Geometry check sheet. Reference: the model listing, model coordinates, mm. A direction names the side the tool comes from. Round coordinates to 2 decimals unless told otherwise and drop trailing zeros. Order: outer loops, then holes, each group sorted by start corner. A loop starts at its lowest first (then second) coordinate and runs counter-clockwise, first axis right, second up. Notation, with made-up numbers: (-11.5, 71) - (-1.5, 71) arc R5 ccw to (-1.5, 75) - close; hole circle Ø1 at (70, 58.25). An arc over 180 degrees is marked (long way). Return JSON: item names as keys, results as strings. Group by question number.
Q1. Gauge pin test, flat ends, axial feed: pin 1 Ø0.6 at (y, z) = (-6.5, 0.5) entering from +X; pin 2 Ø0.5 at (x, z) = (2.5, 1.5) entering from +Y; pin 3 Ø0.8 at (y, z) = (1, 1.5) entering from +X. Record the tip position at first contact, or that the pin passes through.
Q2. Sectioned sample at D-D, the plane x = -6.5. Record the cut outline in (y, z).
Q3. Material ranges on line 1 along Y through (x, z) = (0, 0.8); line 2 along Y through (x, z) = (-11, 0.6) (3 decimals); line 3 along Y through (x, z) = (-5, 1.6), recorded low to high.
Q4. Sectioned sample at C-C, the plane y = 0. Record the cut outline in (x, z).
Q5. Sectioned sample at B-B, the plane x = 0. Record the cut outline in (y, z), then the cut area to 3 significant figures.
Q6. Sectioned sample at A-A, the plane z = 0.3. Record the cut outline in (x, y) (3 decimals).
Q7. Tool access check on faces 1 (the cylindrical face through (-13.15, -5.78, 1.49)), 2 (the cylindrical face through (-12.75, 6.04, 1.49)), 3 (the flat face through (-13.65, -0.2, 1.5)), 4 (the flat face through (0.9, -6.9, 1.5)), 5 (the flat face through (-0.1, 6.9, 1.5)). Record the directions out of +Z, -Z, +X, -X, +Y, -Y that give a thin tool (end or side, any length) a straight path to the whole face; none if there is none.
Q8. Draft check along Y on faces 6 (the flat face through (-8.678, -6, 1)), 7 (the flat face through (3, 3, 2)), 8 (the cylindrical face through (12.79, -6, 1.49)), 9 (the flat face through (-10, -4.875, 1)). Enter one of: pulls with the +Y half, pulls with the -Y half, needs draft (parallel to the pull), parting line crosses it, or undercut.
```python
from build123d import *

# Parameters (mm, degrees)
F0_W        = 30.5
F0_H        = 17
F1_DEPTH    = 1
F2_W        = 27.3
F2_H        = 13.8
F3_DEPTH    = 1
F4_R        = 3.6
F4_W        = 3.1
F4_H        = 2.025
F5_DEPTH    = 2
F6_T1_DEPTH = 7.9496474731
F6_T3_DEPTH = 8.5
F7_R        = 3.5


# Not quite as in the source:
# - a fillet or chamfer that OpenCascade refuses, or shapes differently, is made with other operations: its cross-section is extruded or revolved along the edge and cut away or added


with BuildPart() as f1:
    # F0 (on Top) → F1 (new body)
    with BuildSketch(Plane.XY):
        Rectangle(F0_W, F0_H)
    extrude(amount=F1_DEPTH)

    # F2 (on face) → F3 (join)
    with BuildSketch(Plane.XY.offset(1)):
        Rectangle(F2_W, F2_H)
    extrude(amount=F3_DEPTH)

    # F4 (on face) → F5 (cut)
    with BuildSketch(Plane.XY.offset(2)):
        Circle(F4_R)
        with Locations((-10.228, -5.8875)):
            Rectangle(F4_W, F4_H)
    extrude(amount=-F5_DEPTH, mode=Mode.SUBTRACT)

    # F6: fillet of radius 3 on 4 edges, made by hand

    # F6_s2 → F6_t1 (cut)
    with BuildSketch(Plane.XY.offset(1)):
        with BuildLine():
            ThreePointArc((-13.65, -4.1201410108), (-13.1383729624, -5.795849816), (-11.778, -6.9))
            Line((-11.778, -6.9), (-13.65, -6.9))
            Line((-13.65, -6.9), (-13.65, -4.1201410108))
        make_face()
    extrude(amount=F6_T1_DEPTH, mode=Mode.SUBTRACT)

    # F6_s4 → F6_t3 (cut)
    with BuildSketch(Plane.XY.offset(1)):
        with BuildLine():
            ThreePointArc((13.65, -3.9), (12.7713203436, -6.0213203436), (10.65, -6.9))
            Line((10.65, -6.9), (13.65, -6.9))
            Line((13.65, -6.9), (13.65, -3.9))
        make_face()
        with BuildLine():
            ThreePointArc((-10.65, 6.9), (-12.7713203436, 6.0213203436), (-13.65, 3.9))
            Line((-13.65, 3.9), (-13.65, 6.9))
            Line((-13.65, 6.9), (-10.65, 6.9))
        make_face()
        with BuildLine():
            ThreePointArc((13.65, 3.9), (12.7713203436, 6.0213203436), (10.65, 6.9))
            Line((10.65, 6.9), (13.65, 6.9))
            Line((13.65, 6.9), (13.65, 3.9))
        make_face()
    extrude(amount=F6_T3_DEPTH, mode=Mode.SUBTRACT)

    # F7
    f7_edges = [f1.edges().sort_by_distance(p)[0] for p in [
        (15.25, 8.5, 0.5),
        (-15.25, 8.5, 0.5),
        (-15.25, -8.5, 0.5),
        (15.25, -8.5, 0.5),
    ]]
    fillet(f7_edges, radius=F7_R)


solid = f1.part
```
Reply:
{
 "1": {"pin 1": "x = 15.04", "pin 2": "y = 6.9", "pin 3": "x = 13.65"},
 "2": {"outline": "(-8.5, 0) - (8.5, 0) - (8.5, 1) - (6.9, 1) - (6.9, 2) - (-6.9, 2) - (-6.9, 1) - (-8.5, 1) - close"},
 "3": {"line 1": "-8.5 to -3.6, 3.6 to 8.5", "line 2": "-8.5 to -6.9, -4.875 to 8.5", "line 3": "-6.9 to 6.9"},
 "4": {"outline": "(-15.25, 0) - (-3.6, 0) - (-3.6, 2) - (-13.65, 2) - (-13.65, 1) - (-15.25, 1) - close; (3.6, 0) - (15.25, 0) - (15.25, 1) - (13.65, 1) - (13.65, 2) - (3.6, 2) - close"},
 "5": {"outline": "(-8.5, 0) - (-3.6, 0) - (-3.6, 2) - (-6.9, 2) - (-6.9, 1) - (-8.5, 1) - close; (3.6, 0) - (8.5, 0) - (8.5, 1) - (6.9, 1) - (6.9, 2) - (3.6, 2) - close", "area": "16.4 mm^2"},
 "6": {"outline": "(-15.25, -5) arc R3.5 ccw to (-11.75, -8.5) - (11.75, -8.5) arc R3.5 ccw to (15.25, -5) - (15.25, 5) arc R3.5 ccw to (11.75, 8.5) - (-11.75, 8.5) arc R3.5 ccw to (-15.25, 5) - close; hole (-11.778, -6.9) - (-8.678, -6.9) - (-8.678, -4.875) - (-11.778, -4.875) - close; hole circle Ø7.2 at (0, 0)"},
 "7": {"face 1": "+Z, -X, -Y", "face 2": "+Z, -X, +Y", "face 3": "+Z, -X, +Y, -Y", "face 4": "+Z, +X, -X, -Y", "face 5": "+Z, +X, -X, +Y"},
 "8": {"face 6": "undercut", "face 7": "needs draft", "face 8": "pulls with the -Y half", "face 9": "undercut"}
}
